Model file for the job. Use its own axes, mm. Face numbers are marked on the shaded views. A direction names the side the tool comes from. Coordinates: 2 decimals unless noted, no trailing zeros. Order: outer loops, then holes, each group sorted by start corner. A loop starts at its lowest first (then second) coordinate and runs counter-clockwise, first axis right, second up.
Autodesk Inventor part; units mm, degrees
ref_plane "FDT_PIRODACC_XY" through (0, 0, 34.1) normal (0, 0, 1) x (1, 0, 0)
ref_plane "FDT_PIRODACC_YZ" through (0, 0, 34.1) normal (1, 0, 0) x (0, 1, 0)
ref_plane "FDT_PIRODACC_ZX" through (0, 0, 34.1) normal (0, 1, 0) x (0, 0, 1)
sketch "Sketch_1" plane through (0, 0, 0) normal (1, 0, 0) x (0, 1, 0)
  line L0 (0, -166) -> (0, 25.1)
  line L1 (0, 25.1) -> (5.7172, 25.1)
  line L2 (5.7172, 25.1) -> (6, 24.8172)
  line L3 (6, 24.8172) -> (6, -155.3333)
  line L4 (6, -155.3333) -> (16, -155.3333)
  line L5 (16, -155.3333) -> (16, -166)
  line L6 (16, -166) -> (0, -166)
  line L7 (0, -166) -> (0, 25.1)
revolve "Revolution1" add sketch "Sketch_1" angle 360 about axis through (0, 0, -166) along (0, 0, -1)
sketch "Sketch_2" plane through (0, 0, 0) normal (0, 1, 0) x (-1, 0, 0)
  line L0 (10, 39.1) -> (-10, 39.1)
  line L1 (-10, 39.1) -> (-10, 19.1)
  line L2 (-10, 19.1) -> (-5, 19.1)
  line L3 (-5, 19.1) -> (-5, 31.1)
  line L4 (-5, 31.1) -> (5, 31.1)
  line L5 (5, 31.1) -> (5, 19.1)
  line L6 (5, 19.1) -> (10, 19.1)
  line L7 (10, 19.1) -> (10, 39.1)
extrude "Extrusion1" cut sketch "Sketch_2" along normal mid plane 20
sketch "Sketch_4" plane through (0, 0, 0) normal (1, 0, 0) x (0, 1, 0)
  line L0 (0, 24.5) -> (0, 47.1)
  line L1 (0, 47.1) -> (4.233, 47.1)
  line L2 (4.233, 47.1) -> (5, 46.333)
  line L3 (5, 46.333) -> (5, 29.0727)
  line L4 (5, 29.0727) -> (4.1362, 26.6994)
  arc A0 (4.1362, 26.6994) -> (4.1, 26.4942) centre (4.7, 26.4942) ccw
  line L5 (4.1, 26.4942) -> (4.1, 25.7)
  arc A1 (4.1, 25.7) -> (4.7, 25.1) centre (4.7, 25.7) ccw
  line L6 (4.7, 25.1) -> (4.7, 24.5)
  line L7 (4.7, 24.5) -> (0, 24.5)
  line L8 (0, 24.5) -> (0, 47.1)
revolve "Revolution2" add sketch "Sketch_4" angle 360 about axis through (0, 0, 24.5) along (0, 0, -1)
thread "Thread1"
ref_plane "FDT_PIRODACC_XY" through (0, 0, 34.1) normal (0, 0, 1) x (1, 0, 0)
ref_plane "FDT_PIRODACC_YZ" through (0, 0, 34.1) normal (1, 0, 0) x (0, 1, 0)
ref_plane "FDT_PIRODACC_ZX" through (0, 0, 34.1) normal (0, 1, 0) x (0, 0, 1)
ref_plane "NUT_XY" through (0, 0, 34.1) normal (0, 0, -1) x (1, 0, 0)
ref_plane "NUT_YZ" through (0, 0, 34.1) normal (1, 0, 0) x (0, -1, 0)
ref_plane "NUT_ZX" through (0, 0, 34.1) normal (0, -1, 0) x (0, 0, -1)
ref_plane "P_XY" through (0, 0, -166) normal (0, 0, -1) x (0, 1, 0)
ref_plane "P_YZ" through (0, 0, -166) normal (0, 1, 0) x (1, 0, 0)
ref_plane "P_ZX" through (0, 0, -166) normal (1, 0, 0) x (0, 0, -1)
properties part number "1463250 DSBC-32-100_(K)"
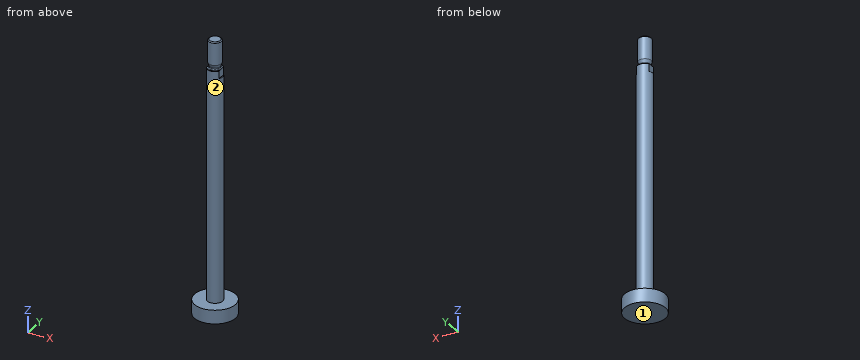
Q1. Cut at C-C, the plane z = -95.5. List the corners of the cut face in (x, y).
Established:
outline: circle Ø12 at (0, 0)
Q2. Cut at A-A, the plane y = 0. List the corners of the cut face in (x, z).
Established:
outline: (-16, -166) - (16, -166) - (16, -155.33) - (6, -155.33) - (6, 19.1) - (5, 19.1) - (5, 25.1) - (4.7, 25.1) arc R0.6 cw to (4.1, 25.7) - (4.1, 26.49) arc R0.6 cw to (4.14, 26.7) - (5, 29.07) - (5, 46.33) - (4.23, 47.1) - (-4.23, 47.1) - (-5, 46.33) - (-5, 29.07) - (-4.14, 26.7) arc R0.6 cw to (-4.1, 26.49) - (-4.1, 25.7) arc R0.6 cw to (-4.7, 25.1) - (-5, 25.1) - (-5, 19.1) - (-6, 19.1) - (-6, -155.33) - (-16, -155.33) - close
Q3. Cut at D-D, the plane y = 10. List the corners of the cut face in (x, z), plus the area to 3 significant figures.
Established:
outline: (-12.49, -166) - (12.49, -166) - (12.49, -155.33) - (-12.49, -155.33) - close
area: 266 mm2
Q4. Cut at B-B, the plane x = 0. List the corners of the cut face in (y, z).
Established:
outline: (-16, -166) - (16, -166) - (16, -155.33) - (6, -155.33) - (6, 24.82) - (5.72, 25.1) - (4.7, 25.1) arc R0.6 cw to (4.1, 25.7) - (4.1, 26.49) arc R0.6 cw to (4.14, 26.7) - (5, 29.07) - (5, 46.33) - (4.23, 47.1) - (-4.23, 47.1) - (-5, 46.33) - (-5, 29.07) - (-4.14, 26.7) arc R0.6 cw to (-4.1, 26.49) - (-4.1, 25.7) arc R0.6 cw to (-4.7, 25.1) - (-5.72, 25.1) - (-6, 24.82) - (-6, -155.33) - (-16, -155.33) - close
Q5. Drop flat-ended pins along their axis: P1, Ø1.1, axis at x = 5.5, y = 0, coming from the +Z side; P2, Ø1.8, axis at y = -1.5, z = 22, coming from the +X side; P3, Ø8, axis at y = -2, z = -96, coming from the -X side. Give the stop position or say it passes through.
Established:
P1: stops at z = 46.38
P2: stops at x = 5
P3: stops at x = -6
Q6. Probe line 1 (X direction, y = -1, z = -156); line 2 (Z direction, x = -10.5, y = -5.5); line 3 (X direction, y = -5, z = -69). List the from-to ranges inside material, lowest first.
Established:
line 1: x = -15.97 to 15.97
line 2: z = -166 to -155.33
line 3: x = -3.32 to 3.32
Q7. Which spindle directions (+Z, -Z, +X, -X, +Y, -Y) get a long thin tool onto all of the face, cutting with end or side? Do the marked faces 1 and 2. Say none if no direction does.
Established:
face 1: -Z, +X, -X, +Y, -Y
face 2: +Z
